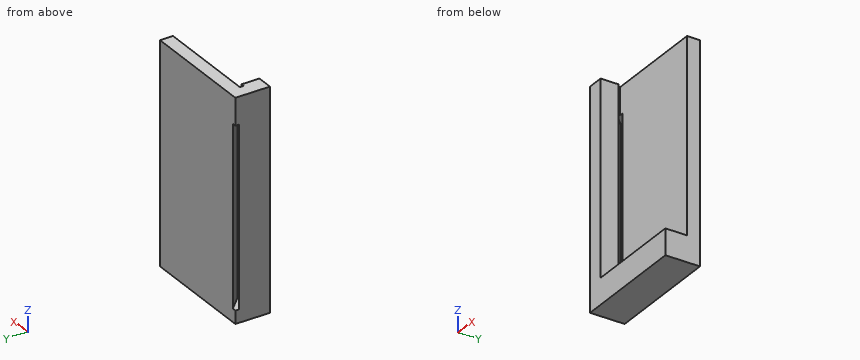
```python
from build123d import *

# Parameters (mm, degrees)
F1_DEPTH = 25
F2_DEPTH = 165
F4_DEPTH = 190
F5_W     = 12
F5_H     = 8
F5_H_2   = 12
F6_DEPTH = 12
F7_W     = 107
F7_H     = 32
F8_DEPTH = 12


with BuildPart() as f1:
    # F0 (on Top) → F1 (new body)
    with BuildSketch(Plane.XY):
        Polygon((-15.4107665035, -11.7272357842), (-11.8752325976, -15.2627696901), (79.5892334965, -15.2627696901), (79.5892334965, -3.2627696901), (-15.4107665035, -3.2627696901), align=None)
        Polygon((-23.8752325976, -3.2627696901), (-15.4107665035, -11.7272357842), (-15.4107665035, -3.2627696901), align=None)
        Polygon((-18.9463004094, -15.2627696901), (-15.4107665035, -15.2627696901), (-27.4107665035, -3.2627696901), (-27.4107665035, -6.7983035961), align=None)
        Polygon((-27.4107665035, -15.2627696901), (-18.9463004094, -15.2627696901), (-27.4107665035, -6.7983035961), align=None)
        Polygon((-15.4107665035, -18.7983035961), (-18.9463004094, -15.2627696901), (-27.4107665035, -15.2627696901), (-27.4107665035, -35.2627696901), (-15.4107665035, -35.2627696901), align=None)
        Polygon((-27.4107665035, -3.2627696901), (-15.4107665035, -15.2627696901), (-15.4107665035, -11.7272357842), (-23.8752325976, -3.2627696901), align=None)
        Polygon((-15.4107665035, -11.7272357842), (-15.4107665035, -15.2627696901), (-11.8752325976, -15.2627696901), align=None)
        Polygon((-15.4107665035, -18.7983035961), (-15.4107665035, -15.2627696901), (-18.9463004094, -15.2627696901), align=None)
    extrude(amount=F1_DEPTH)

    # F0 (on Top) → F2 (join)
    with BuildSketch(Plane.XY):
        Polygon((-15.4107665035, -18.7983035961), (-18.9463004094, -15.2627696901), (-27.4107665035, -15.2627696901), (-27.4107665035, -35.2627696901), (-15.4107665035, -35.2627696901), align=None)
        Polygon((-23.8752325976, -3.2627696901), (-15.4107665035, -11.7272357842), (-15.4107665035, -3.2627696901), align=None)
        Polygon((-15.4107665035, -11.7272357842), (-11.8752325976, -15.2627696901), (79.5892334965, -15.2627696901), (79.5892334965, -3.2627696901), (-15.4107665035, -3.2627696901), align=None)
        Polygon((-27.4107665035, -15.2627696901), (-18.9463004094, -15.2627696901), (-27.4107665035, -6.7983035961), align=None)
    extrude(amount=-F2_DEPTH)

    # F3 (on face) → F4 (join, through all)
    with BuildSketch(Plane(origin=(0, 0, -165), x_dir=(1, 0, 0), z_dir=(0, 0, -1))):
        Polygon((-15.4107665035, 30.7983035961), (-15.4107665035, 18.7983035961), (-12.4107665035, 18.7983035961), (-12.4107665035, 30.7983035961), (-12.4107665035, 35.2627696901), (-15.4107665035, 35.2627696901), align=None)
    extrude(amount=-F4_DEPTH)

    # F5 (on face) → F6 (join)
    with BuildSketch(Plane(origin=(0, 0, -165), x_dir=(1, 0, 0), z_dir=(0, 0, -1))):
        Polygon((-12.4107665035, 35.2627696901), (-12.4107665035, 30.7983035961), (-12.4107665035, 27.2627696901), (67.5892334965, 27.2627696901), (67.5892334965, 35.2627696901), align=None)
        with Locations((73.5892334965, 31.2627696901)):
            Rectangle(F5_W, F5_H)
        with Locations((73.5892334965, 21.2627696901)):
            Rectangle(F5_W, F5_H_2)
        Polygon((79.5892334965, 15.2627696901), (67.5892334965, 15.2627696901), (-11.8752325976, 15.2627696901), (-23.8752325976, 3.2627696901), (79.5892334965, 3.2627696901), align=None)
    extrude(amount=-F6_DEPTH)

    # F7 (on face) → F8 (join)
    with BuildSketch(Plane(origin=(0, 0, -165), x_dir=(1, 0, 0), z_dir=(0, 0, -1))):
        with Locations((26.0892334965, 19.2627696901)):
            Rectangle(F7_W, F7_H)
    extrude(amount=F8_DEPTH)


solid = f1.part
```
Part model, mm, in its own coordinate system. Round coordinates to 2 decimals unless told otherwise and drop trailing zeros. Write each loop counter-clockwise with the first axis right and the second up, starting at its lowest first coordinate (ties: lowest second). Pieces come first, ordered by that corner, then holes. Notation, with made-up numbers: (84, 67) -> (123, 67) arc R8 cw to (123, 82) -> close; hole circle Ø7 at (87.5, 26). An arc over 180 degrees is marked (long way). Return JSON: item names as keys, results as strings. Group by question number.
Q1. Saw through at D-D on y = -9.5. Write the cut outline in (x, z), plus the area to 3 significant figures.
Q2. Pin check, flat tips, straight feed: pin 1 (6 mm diameter, centred on x = 41, y = -28.5, fed in from +Z); pin 2 (1.5 mm diameter, centred on y = -22.5, z = -1, fed in from +X); pin 3 (1 mm diameter, centred on x = 36, y = -24, fed in from +Z). Stop position of each tip, or through.
Q3. Saw through at A-A on z = -122. Write the cut outline in (x, y).
Q4. Saw through at C-C on y = -25. Write the cut outline in (x, z).
Q5. Saw through at B-B on x = 27. Write the cut outline in (y, z), plus the area to 3 significant figures.
Q6. Probe L1, parallel to Z at x = 71.5, y = -21; L2, parallel to X at y = -32.5, z = -94.5; L3, parallel to Y at x = 9, z = -135. List the from-to ranges inside material, lowest first. Write a range as [from, to].
Answer:
{
 "1": {"outline": "(-27.41, -177) -> (79.59, -177) -> (79.59, 25) -> (-27.41, 25) -> close; hole (-24.71, -165) -> (-17.64, -165) -> (-17.64, 0) -> (-24.71, 0) -> close", "area": "20,400 mm2"},
 "2": {"pin 1": "z = -153", "pin 2": "x = -12.41", "pin 3": "z = -165"},
 "3": {"outline": "(-27.41, -35.26) -> (-12.41, -35.26) -> (-12.41, -18.8) -> (-15.41, -18.8) -> (-27.41, -6.8) -> close; (-23.88, -3.26) -> (-11.88, -15.26) -> (79.59, -15.26) -> (79.59, -3.26) -> close"},
 "4": {"outline": "(-27.41, -177) -> (79.59, -177) -> (79.59, -153) -> (67.59, -153) -> (67.59, -165) -> (-12.41, -165) -> (-12.41, 25) -> (-27.41, 25) -> close"},
 "5": {"outline": "(-35.26, -177) -> (-3.26, -177) -> (-3.26, 25) -> (-15.26, 25) -> (-15.26, -165) -> (-27.26, -165) -> (-27.26, -153) -> (-35.26, -153) -> close", "area": "2,760 mm2"},
 "6": {"L1": "[-177, -153]", "L2": "[-27.41, -12.41]", "L3": "[-15.26, -3.26]"}
}
